Check sheet for the modelled part. Datum: model origin and axes. Units: mm. Give positions to 0.01 mm unless a question says otherwise; leave off trailing zeros. Loops run counter-clockwise (first coordinate to the right, second up) from the corner with the lowest first, then second, coordinate; pieces in that order, holes last. Notation, with made-up numbers: M 37.5,23 L 62.5,23 A10 cw 62.5,35 Z; hole C 40,-22.75 d11. An arc over 180 degrees is marked long. Put each result on its own line as item: value. Start each with the question number.
```python
from build123d import *

# Parameters (mm, degrees)
F0_W      = 63.5
F0_H      = 63.5
F0_W_2    = 50.8
F0_H_2    = 50.8
F1_DEPTH  = 165.1
F3_R      = 6.477
F4_DEPTH  = 25.4
F6_DEPTH  = 25.4
F7_R      = 6.35
F8_DEPTH  = 63.501
F9_W      = 145.7979530096
F9_H      = 377.9422044754
F9_W_2    = 50.8
F9_H_2    = 292.1
F10_DEPTH = 63.5
F11_W     = 97.6704657078
F11_H     = 338.8985395432
F12_DEPTH = 57.151


# Not quite as in the source:
# - ends of sketch curves that miss each other by under 0.0002 mm in the source are joined


with BuildPart() as f1:
    # F0 (on Top) → F1 (new body, symmetric)
    with BuildSketch(Plane.XY):
        Rectangle(F0_W, F0_H)
        Rectangle(F0_W_2, F0_H_2, mode=Mode.SUBTRACT)
    extrude(amount=F1_DEPTH, both=True)

    # F3 (on face) → F4 (cut)
    with BuildSketch(Plane.YZ.offset(31.75)):
        with Locations((0, 146.05)):
            Circle(F3_R)
        with BuildLine():
            ThreePointArc((10.1385245046, 129.1766616857), (14.6288058895, 132.8781640138), (17.8406687878, 137.7307595176))
            ThreePointArc((17.8406687878, 137.7307595176), (19.4934269332, 143.3103775076), (19.4426449846, 149.1294124443))
            ThreePointArc((19.4426449846, 149.1294124443), (15.0835370951, 152.2964897102), (11.9164598293, 147.9373818207))
            ThreePointArc((11.9164598293, 147.9373818207), (11.9475842494, 144.3708765369), (10.9346034506, 140.9511106721))
            ThreePointArc((10.9346034506, 140.9511106721), (8.9660423194, 137.9769392343), (6.2139343738, 135.708276517))
            ThreePointArc((6.2139343738, 135.708276517), (4.9104220235, 130.4801740359), (10.1385245046, 129.1766616857))
        make_face()
        with BuildLine():
            ThreePointArc((-10.1385245046, 129.1766616857), (-4.9104220235, 130.4801740359), (-6.2139343738, 135.708276517))
            ThreePointArc((-6.2139343738, 135.708276517), (-8.9660423194, 137.9769392343), (-10.9346034506, 140.9511106721))
            ThreePointArc((-10.9346034506, 140.9511106721), (-11.9475842494, 144.3708765369), (-11.9164598293, 147.9373818207))
            ThreePointArc((-11.9164598293, 147.9373818207), (-15.0835370951, 152.2964897102), (-19.4426449846, 149.1294124443))
            ThreePointArc((-19.4426449846, 149.1294124443), (-19.4934269332, 143.3103775076), (-17.8406687878, 137.7307595176))
            ThreePointArc((-17.8406687878, 137.7307595176), (-14.6288058895, 132.8781640138), (-10.1385245046, 129.1766616857))
        make_face()
    extrude(amount=-F4_DEPTH, mode=Mode.SUBTRACT)

    # F5 (on face) → F6 (cut)
    with BuildSketch(Plane(origin=(-31.75, 0, 0), x_dir=(0, -1, 0), z_dir=(-1, 0, 0))):
        with BuildLine():
            ThreePointArc((-3.1401119103, 140.3850881569), (3.2873259769, 140.4692279278), (6.477, 146.05))
            ThreePointArc((6.477, 146.05), (-3.2873259769, 151.6307720722), (-3.1401119103, 140.3850881569))
        make_face()
        with BuildLine():
            ThreePointArc((-4.5213527214, 132.1654121492), (-4.960680137, 133.7768464516), (-6.1570821771, 134.9423297193))
            ThreePointArc((-6.1570821771, 134.9423297193), (-10.4320253058, 130.5539778468), (-4.5213527214, 132.1654121492))
        make_face()
        with BuildLine():
            ThreePointArc((3.1226517792, 134.3961049058), (0.4285749428, 129.7298269458), (5.0948529028, 127.0357501095))
            ThreePointArc((5.0948529028, 127.0357501095), (17.8406687878, 137.7307595176), (17.8406687878, 154.3692404824))
            ThreePointArc((17.8406687878, 154.3692404824), (12.777460542, 156.2120975737), (10.9346034506, 151.1488893279))
            ThreePointArc((10.9346034506, 151.1488893279), (10.9346034506, 140.9511106721), (3.1226517792, 134.3961049058))
        make_face()
    extrude(amount=-F6_DEPTH, mode=Mode.SUBTRACT)

    # F7 (on face) → F8 (cut, through all)
    with BuildSketch(Plane.YZ.offset(31.75)):
        with BuildLine():
            ThreePointArc((-8.89, 107.949999693), (-15.239999693, 101.6), (-8.89, 95.250000307))
            ThreePointArc((-8.89, 95.250000307), (3.81, 82.55), (-8.89, 69.85))
            ThreePointArc((-8.89, 69.85), (-15.239999693, 63.5), (-8.89, 57.150000307))
            ThreePointArc((-8.89, 57.150000307), (16.509999693, 82.55), (-8.89, 107.949999693))
        make_face()
        with BuildLine():
            ThreePointArc((8.89, 3.07e-07), (15.239999693, 6.35), (8.89, 12.699999693))
            ThreePointArc((8.89, 12.699999693), (-3.81, 25.4), (8.89, 38.1))
            ThreePointArc((8.89, 38.1), (15.24, 44.45), (8.89, 50.8))
            ThreePointArc((8.89, 50.8), (-16.509999693, 25.4), (8.89, 3.07e-07))
        make_face()
        with BuildLine():
            ThreePointArc((-8.89, -6.350000307), (-15.239999693, -12.7), (-8.89, -19.049999693))
            ThreePointArc((-8.89, -19.049999693), (3.81, -31.75), (-8.89, -44.45))
            ThreePointArc((-8.89, -44.45), (-15.239999693, -50.8), (-8.89, -57.149999693))
            ThreePointArc((-8.89, -57.149999693), (16.509999693, -31.75), (-8.89, -6.350000307))
        make_face()
        with BuildLine():
            ThreePointArc((8.89, -114.299999693), (15.239999693, -107.95), (8.89, -101.600000307))
            ThreePointArc((8.89, -101.600000307), (-3.81, -88.9), (8.89, -76.2))
            ThreePointArc((8.89, -76.2), (15.24, -69.85), (8.89, -63.5))
            ThreePointArc((8.89, -63.5), (-16.509999693, -88.9), (8.89, -114.299999693))
        make_face()
        with Locations((-8.89, 82.55)):
            Circle(F7_R)
        with Locations((8.89, 25.4)):
            Circle(F7_R)
        with Locations((8.89, -88.9)):
            Circle(F7_R)
        with Locations((-8.89, -31.75)):
            Circle(F7_R)
    extrude(amount=-F8_DEPTH, mode=Mode.SUBTRACT)

    # F9 (on face) → F10 (cut, symmetric)
    with BuildSketch(Plane(origin=(25.4, 0, 0), x_dir=(0, -1, 0), z_dir=(-1, 0, 0))):
        Rectangle(F9_W, F9_H)
        with Locations((0, 19.05)):
            Rectangle(F9_W_2, F9_H_2, mode=Mode.SUBTRACT)
    extrude(amount=F10_DEPTH, both=True, mode=Mode.SUBTRACT)

    # F11 (on face) → F12 (cut, through all)
    with BuildSketch(Plane.YZ.offset(-25.4)):
        Rectangle(F11_W, F11_H)
    extrude(amount=F12_DEPTH, mode=Mode.SUBTRACT)


solid = f1.part
```
Q1. Mould release check, pull along Z, two halves, no side actions. Record for faces 1 (the face through (-28.62, -0.41, 129.81)), 2 (the face through (-29, 0, -127)), 3 (the face through (-29, 0, 165.1)): pulls with the +Z half, pulls with the -Z half, needs draft (parallel to the pull), parting line crosses it, or undercut.
Q2. Thickness scan on line 1 along Y through (x, z) = (-28.5, 143.5); line 2 along Y through (x, z) = (-29.25, 134); line 3 along Y through (x, z) = (-28.25, 64). Record the ranges inside material, lowest first. Write a range as [from, to].
Q3. Section check B-B, the plane z = 82.55. Record the cut outline in (x, y).
Q4. Section check A-A, the plane z = 41.5. Record the cut outline in (x, y), then the cut area to 3 significant figures.
Q5. Depth check by flat-ended pin: P1, Ø10, axis at y = -8.89, z = -31.75, coming from the -X side (3 decimals). Enter the tip coordinate at first touch or a pass-through.
Q6. Section check C-C, the plane x = -29.5. Give the number of separate pieces and of enclosed holes in the cut face, then the cut area to 3 significant figures.
Found:
1. face 1: undercut
1. face 2: pulls with the -Z half
1. face 3: pulls with the +Z half
2. line 1: y = [-25.4, -19.52], [-11.79, -5.95], [5.95, 25.4]
2. line 2: y = [-25.4, -15.57], [-2.18, 5.11], [10.29, 25.4]
2. line 3: y = [-25.4, -15.22], [8.46, 25.4]
3. outline: M -31.75,-25.4 L -25.4,-25.4 L -25.4,-15.24 L -31.75,-15.24 Z; M -31.75,-2.54 L -25.4,-2.54 L -25.4,3.81 L -31.75,3.81 Z; M -31.75,16.51 L -25.4,16.51 L -25.4,25.4 L -31.75,25.4 Z
4. outline: M -31.75,-25.4 L -25.4,-25.4 L -25.4,-10.76 L -31.75,-10.76 Z; M -31.75,14.51 L -25.4,14.51 L -25.4,25.4 L -31.75,25.4 Z
4. area: 162 mm^2
5. P1: passes through
6. separate pieces: 1
6. enclosed holes: 11
6. area: 10,400 mm^2
